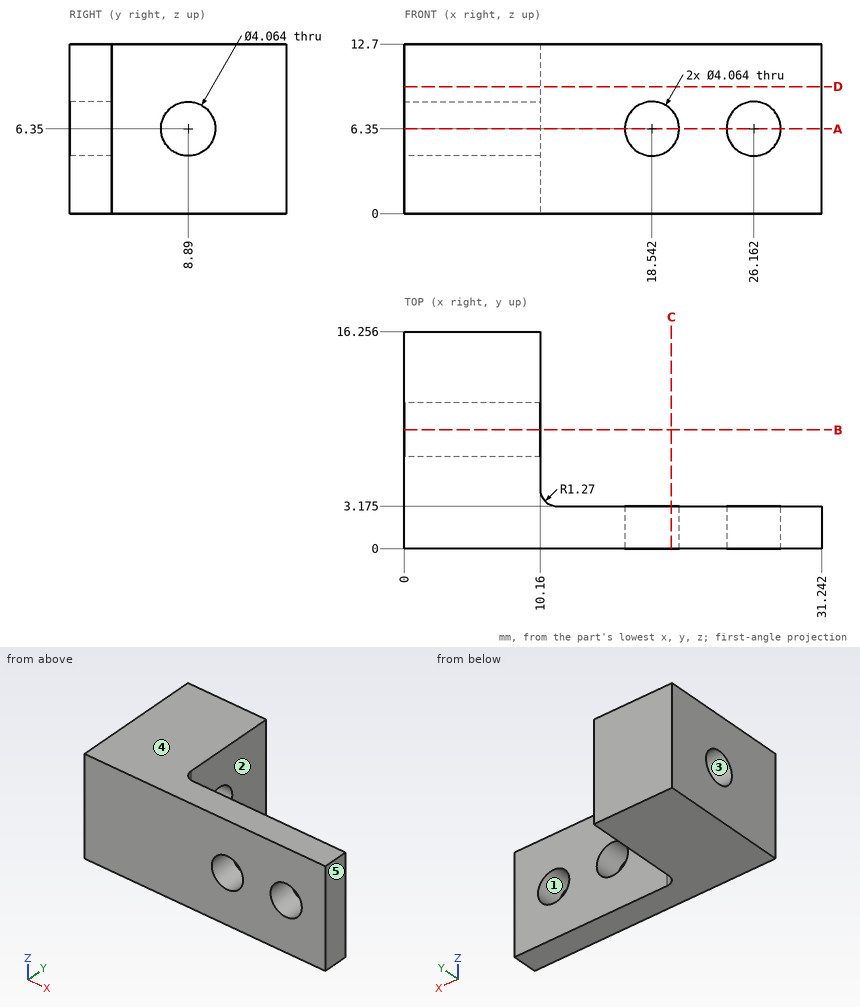
Verification items for this drawing (mm, ordinates from the low corner). A direction names the side the tool comes from. Give positions to 0.01 mm unless a question says otherwise; leave off trailing zeros. Write each loop counter-clockwise with the first axis right and the second up, starting at its lowest first coordinate (ties: lowest second). Pieces come first, ordered by that corner, then holes. Notation, with made-up numbers: (9, 48) - (53, 48) arc R24 ccw to (53, 71) - close; hole circle Ø5 at (38, -32.5). An arc over 180 degrees is marked (long way). Answer as a JSON object with one key per item and string values. Group by question number.
1) Sectioned sample at C-C (x = 20). Record the cut outline in (y, z) (3 decimals).
2) Sectioned sample at B-B (y = 8.89). Record the cut outline in (x, z), then the cut area to 3 significant figures.
3) Thickness scan on probe 1 along Y at (x, z) = (5.25, 6.35); probe 2 along Y at (x, z) = (13.5, 7.25) (3 decimals); probe 3 along X at (y, z) = (14.25, 3.25). Record the ranges inside material, lowest first. Write a range as from..to.
4) Sectioned sample at D-D (z = 9.5). Record the cut outline in (x, y) (3 decimals).
5) Access from +Z, -Z, +X, -X, +Y, -Y to the whole of each face (thin tool, end or side, straight path). Record for the marked faces 1 and 2.
6) Release check for a two-part mould opening along Z. For the marked faces 3, 4 and 5 record: pulls with the +Z half, pulls with the -Z half, needs draft (parallel to the pull), parting line crosses it, or undercut.
7) Depth check by flat-ended pin: P1, Ø3.5, axis at y = 8.89, z = 6.35, coming from the +X side; P2, Ø1, axis at x = 21.5, z = 10.5, coming from the +Y side (3 decimals); P3, Ø3.5, axis at y = 11, z = 9.5, coming from the +X side. Enter the tip coordinate at first touch or a pass-through.
8) Sectioned sample at A-A (z = 6.35). Record the cut outline in (x, y) (3 decimals).
Geometry results:
{
 "1": {"outline": "(0, 0) - (3.175, 0) - (3.175, 4.935) - (0, 4.935) - close; (0, 7.765) - (3.175, 7.765) - (3.175, 12.7) - (0, 12.7) - close"},
 "2": {"outline": "(0, 0) - (10.16, 0) - (10.16, 4.32) - (0, 4.32) - close; (0, 8.38) - (10.16, 8.38) - (10.16, 12.7) - (0, 12.7) - close", "area": "87.7 mm^2"},
 "3": {"probe 1": "y = 0..6.86, 10.92..16.26", "probe 2": "y = 0..3.175", "probe 3": "x = 0..10.16"},
 "4": {"outline": "(0, 0) - (31.242, 0) - (31.242, 3.175) - (11.43, 3.175) arc R1.27 cw to (10.16, 4.445) - (10.16, 16.256) - (0, 16.256) - close"},
 "5": {"face 1": "+Y, -Y", "face 2": "+Z, -Z, +X, +Y"},
 "6": {"face 3": "undercut", "face 4": "pulls with the +Z half", "face 5": "needs draft"},
 "7": {"P1": "passes through", "P2": "stops at y = 3.175", "P3": "stops at x = 10.16"},
 "8": {"outline": "(0, 0) - (16.51, 0) - (16.51, 3.175) - (11.43, 3.175) arc R1.27 cw to (10.16, 4.445) - (10.16, 6.858) - (0, 6.858) - close; (0, 10.922) - (10.16, 10.922) - (10.16, 16.256) - (0, 16.256) - close; (20.574, 0) - (24.13, 0) - (24.13, 3.175) - (20.574, 3.175) - close; (28.194, 0) - (31.242, 0) - (31.242, 3.175) - (28.194, 3.175) - close"}
}
